Geometry: final body of the model. Coordinates: model frame, mm. Face numbers are marked on the shaded views. A direction names the side the tool comes from. Give positions to 0.01 mm unless a question says otherwise; leave off trailing zeros. Write each loop counter-clockwise with the first axis right and the second up, starting at its lowest first coordinate (ties: lowest second). Pieces come first, ordered by that corner, then holes.
```python
from build123d import *

# Parameters (mm, degrees)
SKETCH1_R           = 0.8449945
SKETCH1_W           = 19.05
SKETCH1_H           = 6.0000896
SKETCH1_W_2         = 6.35
SKETCH1_H_2         = 6.35
BOSS_EXTRUDE1_DEPTH = 6.35
FILLET3_R           = 1


with BuildPart() as part:
    # Sketch1 → Boss-Extrude1 (new body)
    with BuildSketch(Plane(origin=(0, 0, 0), x_dir=(1, 0, 0), z_dir=(0, 1, 0))):
        Polygon((0, 14.393729658), (0, 6.0000896), (3.5249993, 6.0000896), (3.5249993, 12.728734258), (3.5249993, 14.393729658), align=None)
        with Locations((1.88250068, 12.728734258)):
            Circle(SKETCH1_R, mode=Mode.SUBTRACT)
        with BuildLine():
            Line((3.5249993, 12.728734258), (3.5249993, 6.0000896))
            Line((3.5249993, 6.0000896), (15.5250007, 6.0000896))
            Line((15.5250007, 6.0000896), (15.5250007, 12.7287274))
            ThreePointArc((15.5250007, 12.7287274), (9.524996571, 6.7287267), (3.5249993, 12.728734258))
        make_face()
        Polygon((15.5250007, 12.7287274), (15.5250007, 6.0000896), (19.05, 6.0000896), (19.05, 14.393729658), (15.5250007, 14.393729658), align=None)
        with Locations((17.16749932, 12.7287274)):
            Circle(SKETCH1_R, mode=Mode.SUBTRACT)
        with Locations((9.525, 3.0000448)):
            Rectangle(SKETCH1_W, SKETCH1_H)
        with Locations((3.175, -3.175)):
            Rectangle(SKETCH1_W_2, SKETCH1_H_2)
        with Locations((15.875, -3.175)):
            Rectangle(SKETCH1_W_2, SKETCH1_H_2)
    extrude(amount=BOSS_EXTRUDE1_DEPTH)

    # Fillet3
    fillet3_edges = [part.edges().sort_by_distance(p)[0] for p in [
        (19.05, 3.175, 6.35),
        (12.7, 3.175, 6.35),
        (6.35, 3.175, 6.35),
        (0, 3.175, 6.35),
        (0, 3.175, -14.393729658),
        (3.5249993, 3.175, -14.393729658),
        (15.5250007, 3.175, -14.393729658),
        (19.05, 3.175, -14.393729658),
    ]]
    fillet(fillet3_edges, radius=FILLET3_R)


solid = part.part
```
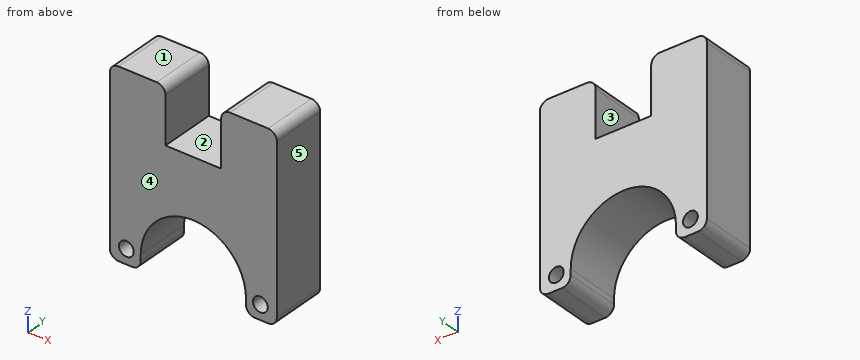
Item 1: Section D-D, the plane x = 11.5. Return the cut outline in (y, z).
Found:
outline: (0, -7.06) - (6.35, -7.06) - (6.35, 0) - (0, 0) - close
Item 2: Section A-A, the plane y = 1.5. State how many separate pieces and enclosed holes the cut face has, plus the area to 3 significant figures.
Found:
separate pieces: 1
enclosed holes: 2
area: 272 mm2
Item 3: Pull-direction query (X, two-part tool) for the marked faces 3, 4 and 5; classes: +X half, -X half, draft (parallel to the pull), parting line (faces both ways), or undercut.
Found:
face 3: undercut
face 4: draft
face 5: +X half
Item 4: Line query: L1, parallel to X at y = 4.25, z = 2.75; L2, parallel to Z at x = 9.5, y = 4.5; L3, parallel to X at y = 4.25, z = -7.75. Output: solid intervals per line, ascending.
Found:
L1: x = 0 to 6.35, 12.7 to 19.05
L2: z = -6.73 to 0
L3: x = 0 to 6.18, 12.87 to 19.05
Item 5: Section B-B, the plane z = 4.75. Return the cut outline in (x, y), plus the area to 3 significant figures.
Found:
outline: (0, 0) - (6.35, 0) - (6.35, 6.35) - (0, 6.35) - close; (12.7, 0) - (19.05, 0) - (19.05, 6.35) - (12.7, 6.35) - close
area: 80.6 mm2
Item 6: Section C-C, the plane x = 2. Return the cut outline in (y, z).
Found:
outline: (0, -14.39) - (6.35, -14.39) - (6.35, -13.57) - (0, -13.57) - close; (0, -11.89) - (6.35, -11.89) - (6.35, 6.35) - (0, 6.35) - close
Item 7: Reachability of the marked faces 1 and 2 from +Z, -Z, +X, -X, +Y, -Y: full face, straight path, thin tool, end or side. Return the list, or none.
Found:
face 1: +Z, +X, -X, +Y, -Y
face 2: +Z, +Y, -Y
